Autodesk Inventor part; units mm, degrees
ref_plane "CP1_XY" through (0, 0, -84.4) normal (0, 0, -1) x (1, 0, 0)
ref_plane "CP1_YZ" through (0, 0, -84.4) normal (1, 0, 0) x (0, -1, 0)
ref_plane "CP1_ZX" through (0, 0, -84.4) normal (0, -1, 0) x (0, 0, -1)
sketch "Sketch_1" plane through (0, 0, 0) normal (1, 0, 0) x (0, 1, 0)
  line L0 (0, -84.4) -> (0, 0)
  line L1 (0, 0) -> (3, 0)
  line L2 (3, 0) -> (3, -79.4)
  line L3 (3, -79.4) -> (8, -79.4)
  line L4 (8, -79.4) -> (8, -84.4)
  line L5 (8, -84.4) -> (0, -84.4)
  line L6 (0, -84.4) -> (0, 0)
revolve "Revolution1" add sketch "Sketch_1" angle 360 about axis through (0, 0, -84.4) along (0, 0, -1)
sketch "Sketch_2" plane through (0, 0, 0) normal (1, 0, 0) x (0, 1, 0)
  line L0 (0, 0) -> (0, 12)
  line L1 (0, 12) -> (2.3865, 12)
  line L2 (2.3865, 12) -> (3, 11.3865)
  line L3 (3, 11.3865) -> (3, 2.2222)
  line L4 (3, 2.2222) -> (2.0586, 1.2808)
  arc A0 (2.0586, 1.2808) -> (2, 1.1394) centre (2.2, 1.1394) ccw
  line L5 (2, 1.1394) -> (2, 0.2)
  arc A1 (2, 0.2) -> (2.2, 0) centre (2.2, 0.2) ccw
  line L6 (2.2, 0) -> (0, 0)
  line L7 (0, 0) -> (0, 12)
revolve "Revolution2" add sketch "Sketch_2" angle 360 about axis through (0, 0, 0) along (0, 0, -1)
thread "Thread1"
sketch "Sketch_8" plane through (0, 0, 0) normal (0, 0, 1) x (1, 0, 0)
  line L0 (-4.5, 5) -> (-4.5, -5)
  line L1 (-4.5, -5) -> (4.5, -5)
  line L2 (4.5, -5) -> (4.5, 5)
  line L3 (4.5, 5) -> (-4.5, 5)
  line L4 (-2.5, -4) -> (2.5, -4)
  line L5 (2.5, -4) -> (2.5, 4)
  line L6 (2.5, 4) -> (-2.5, 4)
  line L7 (-2.5, 4) -> (-2.5, -4)
extrude "Extrusion1" cut sketch "Sketch_8" against normal blind 3
ref_plane "CP1_XY" through (0, 0, -84.4) normal (0, 0, -1) x (1, 0, 0)
ref_plane "CP1_YZ" through (0, 0, -84.4) normal (1, 0, 0) x (0, -1, 0)
ref_plane "CP1_ZX" through (0, 0, -84.4) normal (0, -1, 0) x (0, 0, -1)
ref_plane "CP_P_XY" through (0, 0, -84.4) normal (0, 0, 1) x (1, 0, 0)
ref_plane "CP_P_YZ" through (0, 0, -84.4) normal (1, 0, 0) x (0, 1, 0)
ref_plane "CP_P_ZX" through (0, 0, -84.4) normal (0, 1, 0) x (0, 0, 1)
ref_plane "CP_PL_XY" through (0, 0, -3) normal (0, 0, 1) x (1, 0, 0)
ref_plane "CP_PL_YZ" through (0, 0, -3) normal (1, 0, 0) x (0, 1, 0)
ref_plane "CP_PL_ZX" through (0, 0, -3) normal (0, 1, 0) x (0, 0, 1)
ref_plane "DIM_ZM_XY" through (0, 3, -157) normal (1, 0, 0) x (0, 0, -1)
ref_plane "DIM_ZM_YZ" through (0, 3, -157) normal (0, 0, -1) x (0, 1, 0)
ref_plane "DIM_ZM_ZX" through (0, 3, -157) normal (0, 1, 0) x (1, 0, 0)
ref_plane "DISC_XY" through (0, 0, 5) normal (0, 0, -1) x (1, 0, 0)
ref_plane "DISC_YZ" through (0, 0, 5) normal (1, 0, 0) x (0, -1, 0)
ref_plane "DISC_ZX" through (0, 0, 5) normal (0, -1, 0) x (0, 0, -1)
ref_plane "NUT_6_10_T_1_XY" through (0, 0, -168) normal (0, 0, 1) x (1, 0, 0)
ref_plane "NUT_6_10_T_1_YZ" through (0, 0, -168) normal (1, 0, 0) x (0, 1, 0)
ref_plane "NUT_6_10_T_1_ZX" through (0, 0, -168) normal (0, 1, 0) x (0, 0, 1)
ref_plane "NUT_6_10_T_2_XY" through (0, 0, -165.8) normal (0, 0, 1) x (1, 0, 0)
ref_plane "NUT_6_10_T_2_YZ" through (0, 0, -165.8) normal (1, 0, 0) x (0, 1, 0)
ref_plane "NUT_6_10_T_2_ZX" through (0, 0, -165.8) normal (0, 1, 0) x (0, 0, 1)
ref_plane "NUT_CP_6_10_1_XY" through (0, 0, 10) normal (0, 0, 1) x (1, 0, 0)
ref_plane "NUT_CP_6_10_1_YZ" through (0, 0, 10) normal (1, 0, 0) x (0, 1, 0)
ref_plane "NUT_CP_6_10_1_ZX" through (0, 0, 10) normal (0, 1, 0) x (0, 0, 1)
ref_plane "NUT_CP_6_10_2_XY" through (0, 0, 7.8) normal (0, 0, 1) x (1, 0, 0)
ref_plane "NUT_CP_6_10_2_YZ" through (0, 0, 7.8) normal (1, 0, 0) x (0, 1, 0)
ref_plane "NUT_CP_6_10_2_ZX" through (0, 0, 7.8) normal (0, 1, 0) x (0, 0, 1)
properties part number "4186566 DPDM-Q-50---(r)"
For this review, take the finished solid that the model builds, in its own axes (mm). A direction names the side the tool comes from. Give positions to 0.01 mm unless a question says otherwise; leave off trailing zeros. Loops run counter-clockwise (first coordinate to the right, second up) from the corner with the lowest first, then second, coordinate; pieces in that order, holes last. Notation, with made-up numbers: M -9,21.5 L 1,21.5 A16 cw 1,36.5 Z; hole C 31,-30.75 d3. An arc over 180 degrees is marked long. One line per item, written item: value. Start each with the question number.
Q1. Machinability: for faces 1 (the face through (-2.5, 0, -1)), 2 (the face through (0, -3, 7)), 3 (the face through (2.3, 0.6, 0)), which of the approach directions +Z, -Z, +X, -X, +Y, -Y give a long, thin tool a straight path to every point of the face, cutting with its end or side? Answer none if there is none.
Q2. Add section A-A (y = 0). Give the boundary of the cut face in (x, z), and give its area (3 significant figures).
Q3. Add section B-B (x = 0). Give the boundary of the cut face in (y, z).
Q4. Clearance check with flat-ended pins moving along their axes: pin 1 Ø0.6 at (x, y) = (-3, 0) entering from +Z; pin 2 Ø3.5 at (y, z) = (-0.5, -1) entering from +X; pin 3 Ø2.5 at (y, z) = (0, -1) entering from -X. State where each tip first meets the part, or that it passes through.
Q5. Draft analysis for pull direction Z (two halves, no side actions). For faces 4 (the face through (2.5, 0, -1)), 5 (the face through (0.1, 3.4, -79.4)), 6 (the face through (0, 0, -84.4)), 7 (the face through (-1.952, -0.434, 0.663)), state which applies: released by +Z, released by -Z, zero draft, split by the parting line, or undercut.
Q6. Add section D-D (y = 5.25). Give the boundary of the cut face in (x, z).
Q7. For L1, parallel to Z at x = -6, y = -2; L2, parallel to Y at x = -2.25, z = -6; L3, parallel to Y at x = 2.5, z = -32, list the stretches that pass through material, from the lowest coordinate up.
Q8. Add section C-C (z = -62). Give the boundary of the cut face in (x, y), and give its area (3 significant figures).
Reply:
1. face 1: -X, +Y, -Y
1. face 2: +Z
1. face 3: none
2. outline: M -8,-84.4 L 8,-84.4 L 8,-79.4 L 3,-79.4 L 3,-3 L 2.5,-3 L 2.5,0 L 2.2,0 A0.2 cw 2,0.2 L 2,1.14 A0.2 cw 2.06,1.28 L 3,2.22 L 3,11.39 L 2.39,12 L -2.39,12 L -3,11.39 L -3,2.22 L -2.06,1.28 A0.2 cw -2,1.14 L -2,0.2 A0.2 cw -2.2,0 L -2.5,0 L -2.5,-3 L -3,-3 L -3,-79.4 L -8,-79.4 Z
2. area: 622 mm²
3. outline: M -8,-84.4 L 8,-84.4 L 8,-79.4 L 3,-79.4 L 3,0 L 2.2,0 A0.2 cw 2,0.2 L 2,1.14 A0.2 cw 2.06,1.28 L 3,2.22 L 3,11.39 L 2.39,12 L -2.39,12 L -3,11.39 L -3,2.22 L -2.06,1.28 A0.2 cw -2,1.14 L -2,0.2 A0.2 cw -2.2,0 L -3,0 L -3,-79.4 L -8,-79.4 Z
4. pin 1: z = 11.69
4. pin 2: x = 2.5
4. pin 3: x = -2.5
5. face 4: undercut
5. face 5: released by +Z
5. face 6: released by -Z
5. face 7: undercut
6. outline: M -6.04,-84.4 L 6.04,-84.4 L 6.04,-79.4 L -6.04,-79.4 Z
7. L1: -84.4 to -79.4
7. L2: -1.98 to 1.98
7. L3: -1.66 to 1.66
8. outline: C 0,0 d6
8. area: 28.3 mm²
